```python
from build123d import *

# Parameters (mm, degrees)
BOSS_EXTRUDE1_DEPTH = 11.90625
SKETCH2_W           = 33.274
SKETCH2_H           = 381
CUT_EXTRUDE1_DEPTH  = 12.90625


with BuildPart() as part:
    # Sketch1 → Boss-Extrude1 (new body)
    with BuildSketch(Plane.XY):
        with BuildLine():
            Line((-101.285966724, 306.196742645), (0.115853822, 306.196742645))
            Line((0.115853822, 306.196742645), (20.943853822, 306.196742645))
            Line((20.943853822, 306.196742645), (20.943853822, 111.886742645))
            Line((20.943853822, 111.886742645), (20.943853822, 34.495334159))
            Line((20.943853822, 34.495334159), (20.943853822, 17.413022699))
            Line((20.943853822, 17.413022699), (127.616425214, 8.080381993))
            ThreePointArc((127.616425214, 8.080381993), (137.378567656, 4.036770195), (141.422179454, -5.725372247))
            Line((141.422179454, -5.725372247), (141.422179454, -74.803257355))
            Line((141.422179454, -74.803257355), (133.664033276, -74.803257355))
            Line((133.664033276, -74.803257355), (-101.285966724, -74.803257355))
            Line((-101.285966724, -74.803257355), (-101.285966724, 306.196742645))
        make_face()
    extrude(amount=BOSS_EXTRUDE1_DEPTH)

    # Sketch2 → Cut-Extrude1 (cut, through all)
    with BuildSketch(Plane.XY.offset(11.90625)):
        with Locations((-84.648966724, 115.696742645)):
            Rectangle(SKETCH2_W, SKETCH2_H)
    extrude(amount=-CUT_EXTRUDE1_DEPTH, mode=Mode.SUBTRACT)


solid = part.part
```
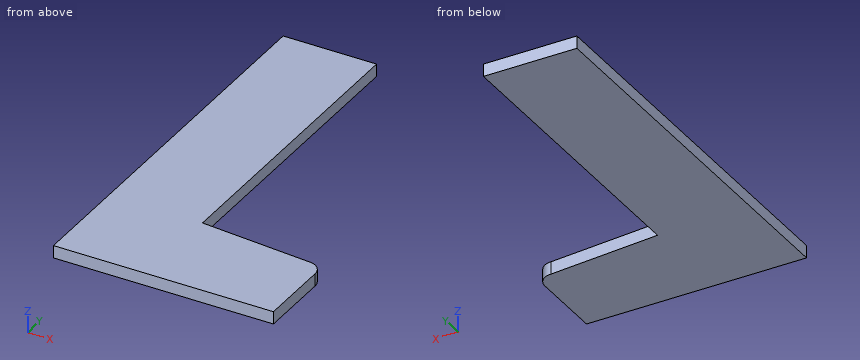
Part model, mm, in its own coordinate system. Coordinates: 2 decimals unless noted, no trailing zeros. Loops run counter-clockwise (first coordinate to the right, second up) from the corner with the lowest first, then second, coordinate; pieces in that order, holes last. Notation, with made-up numbers: (-12, 75) - (-6, 75) arc R18 ccw to (-6, 102) - close; hole circle Ø3 at (3, -27). An arc over 180 degrees is marked (long way). Write item = value, one per line. Start each with the question number.
Item 1: Wall check: L1, parallel to X at y = 71, z = 10.25; L2, parallel to Y at x = 109, z = 1.25; L3, parallel to X at y = -4, z = 10. Give the ranges that are in metal, low to high. Write a range as from..to.
Item 2: Flat gauge pins, fed straight in: pin 1 Ø6 at (y, z) = (234, 8) entering from +X; pin 2 Ø4 at (x, z) = (53, 6.5) entering from +Y; pin 3 Ø5 at (x, z) = (98, 1.5) entering from +Y. Where does each tip first touch, or does it go through?
Item 3: Cut at B-B, the plane y = 113. Give the cut face in (x, z).
Item 4: Cut at C-C, the plane x = 100.5. Give the cut face in (y, z), and give its area (3 significant figures).
Item 5: Cut at A-A, the plane z = 5. Give the cut face in (x, y), and give its area (3 significant figures).
The answers:
q1.L1 = -68.01..20.94
q1.L2 = -74.8..9.71
q1.L3 = -68.01..141.31
q2.pin_1 = 20.94
q2.pin_2 = 14.78
q2.pin_3 = 10.89
q3.outline = (-68.01, 0) - (20.94, 0) - (20.94, 11.91) - (-68.01, 11.91) - close
q4.outline = (-74.8, 0) - (10.45, 0) - (10.45, 11.91) - (-74.8, 11.91) - close
q4.area = 1,020 mm2
q5.outline = (-68.01, -74.8) - (141.42, -74.8) - (141.42, -5.73) arc R13.81 ccw to (127.62, 8.08) - (20.94, 17.41) - (20.94, 306.2) - (-68.01, 306.2) - close
q5.area = 44,300 mm2
